Read the model definition and answer for the solid it produces. Units are mm, in the model's axes. Face numbers are marked on the shaded views. A direction names the side the tool comes from. Coordinates: 2 decimals unless noted, no trailing zeros. Order: outer loops, then holes, each group sorted by start corner. A loop starts at its lowest first (then second) coordinate and runs counter-clockwise, first axis right, second up. Notation, with made-up numbers: (31.5, 12) - (37.5, 12) arc R16 ccw to (37.5, 32) - close; hole circle Ø4 at (52, -26.5). An arc over 180 degrees is marked (long way). Use one line per item in the form item = value. Start each with the question number.
from build123d import *

# Parameters (mm, degrees)
F0_W = 31.75
F0_H = 9.525
F2_W = 25.4
F2_H = 7.9375


with BuildPart() as f1:
    # F0 (on Front) → F1 (revolve)
    with BuildSketch(Plane.XZ):
        with Locations((-41.275, 4.7625)):
            Rectangle(F0_W, F0_H)
        Polygon((-25.4, 9.525), (-25.4, 0), (-12.7, 0), (-12.7, 38.89375), (-12.7, 46.83125), (-12.7, 50.8), (-25.4, 50.8), align=None)
    revolve(axis=Axis((-41.275, 0, 0), (-1, 0, 0)))



with BuildPart() as f1b:
    # F0 (on Front) → F1, piece 2 (revolve)
    with BuildSketch(Plane.XZ):
        Polygon((12.7, 46.83125), (12.7, 38.89375), (12.7, 0), (25.4, 0), (25.4, 9.525), (25.4, 50.8), (12.7, 50.8), align=None)
        with Locations((41.275, 4.7625)):
            Rectangle(F0_W, F0_H)
    revolve(axis=Axis((-41.275, 0, 0), (-1, 0, 0)))


with BuildPart() as f1_1:
    add(f1.part)

    add(f1b.part)  # F3 merges F1b
    # F2 (on Front) → F3 (revolve)
    with BuildSketch(Plane.XZ):
        with Locations((0, 42.8625)):
            Rectangle(F2_W, F2_H)
    revolve(axis=Axis((0, 0, 38.89375), (1, 0, 0)))


solid = f1_1.part
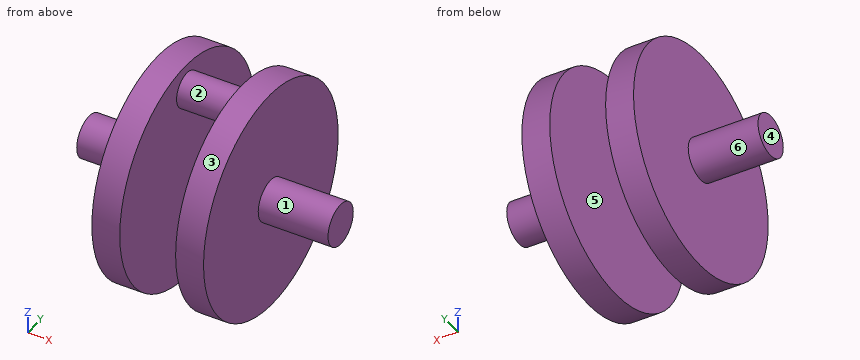
Q1. Which of the six approach directions +Z, -Z, +X, -X, +Y, -Y give full straight-line access (tool end or side, diameter ignored) to the marked faces 1, 2 and 3?
Q2. A cutting plane is placed at A-A (z = 0). Give the vertices of the cut face in (x, y) (3 decimals), then the cut area to 3 significant figures.
Q3. A cutting plane is placed at C-C (y = 0). Give the vertices of the cut face in (x, z) (3 decimals), then the cut area to 3 significant figures.
Q4. For a pull along X with two mould halves and no side action, classify the marked faces 4, 5 and 6 as +X half, -X half, draft (parallel to the pull), parting line (faces both ways), or undercut.
Q5. Consider probe 1 along X at (y, z) = (29, 3); probe 2 along Z at (x, y) = (-18.5, 21); probe 3 along Y at (x, z) = (21, -32). Determine where each line is inside the solid, lowest interval first.
Q6. A cutting plane is placed at B-B (y = 30). Give the vertices of the cut face in (x, z).
Q7. Given P1, Ø1.5, axis at x = 18, y = 26, coming from the +Z side; P2, Ø8, axis at x = 25, z = 22.5, coming from the +Y side; P3, Ø8, axis at y = 36, z = 12, coming from the -X side; P4, Ø10, axis at x = 41.5, y = 17.5, coming from the +Z side, each flat-ended and moving along its own axis, determine where each tip first touches the part or whether it passes through.
Q8. A cutting plane is placed at D-D (x = -0.5). Give the vertices of the cut face in (y, z) (1 decimal), then the cut area to 3 significant figures.
Result sheet:
q1.face_1 = +X
q1.face_2 = none
q1.face_3 = +X, -X
q2.outline = (-57.15, -9.525) - (-25.4, -9.525) - (-25.4, -50.8) - (-12.7, -50.8) - (-12.7, 50.8) - (-25.4, 50.8) - (-25.4, 9.525) - (-57.15, 9.525) - close; (12.7, -50.8) - (25.4, -50.8) - (25.4, -9.525) - (57.15, -9.525) - (57.15, 9.525) - (25.4, 9.525) - (25.4, 50.8) - (12.7, 50.8) - close
q2.area = 3,790 mm^2
q3.outline = (-57.15, -9.525) - (-25.4, -9.525) - (-25.4, -50.8) - (-12.7, -50.8) - (-12.7, 30.956) - (12.7, 30.956) - (12.7, -50.8) - (25.4, -50.8) - (25.4, -9.525) - (57.15, -9.525) - (57.15, 9.525) - (25.4, 9.525) - (25.4, 50.8) - (12.7, 50.8) - (12.7, 46.831) - (-12.7, 46.831) - (-12.7, 50.8) - (-25.4, 50.8) - (-25.4, 9.525) - (-57.15, 9.525) - close
q3.area = 4,190 mm^2
q4.face_4 = -X half
q4.face_5 = undercut
q4.face_6 = draft
q5.probe_1 = -25.4 to -12.7, 12.7 to 25.4
q5.probe_2 = -46.26 to 46.26
q5.probe_3 = -39.45 to 39.45
q6.outline = (-25.4, -41) - (-12.7, -41) - (-12.7, 41) - (-25.4, 41) - close; (12.7, -41) - (25.4, -41) - (25.4, 41) - (12.7, 41) - close
q7.P1 = 44.08
q7.P2 = 47.31
q7.P3 = -25.4
q7.P4 = through
q8.outline = circle Ø15.9 at (0, 38.9)
q8.area = 198 mm^2
